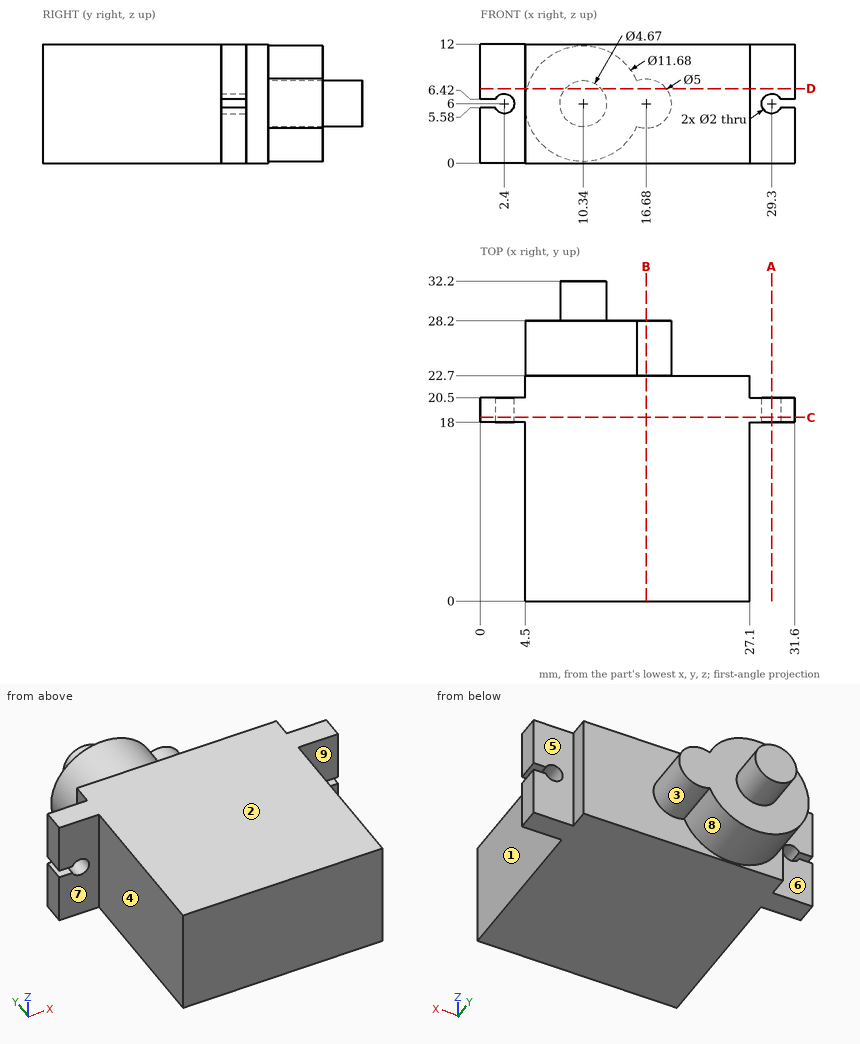
Study the drawing (mm; zero at the part's minimum x, y, z) and answer. A direction names the side the tool comes from. Give positions to 0.01 mm unless a question says otherwise; leave off trailing zeros. Write each loop counter-clockwise with the first axis right and the second up, starting at its lowest first coordinate (ties: lowest second). Pieces come first, ordered by that corner, then holes. Notation, with made-up numbers: (45.25, 76) -> (69.25, 76) arc R22 ccw to (69.25, 97) -> close; hole circle Ø6 at (1, -30.5). An arc over 180 degrees is marked (long way). Write item = value, one per line. Start each with the question number.
1) The part is cut by section A-A, the plane x = 29.3. Determine the outline of the cut face in (y, z).
2) Which of the six approach directions +Z, -Z, +X, -X, +Y, -Y give full straight-line access (tool end or side, diameter ignored) to the marked faces 5, 6, 7, 8 and 9?
3) The part is cut by section D-D, the plane z = 7.5. Determine the outline of the cut face in (x, y), and give its area (3 significant figures).
4) The part is cut by section C-C, the plane y = 18.5. Determine the outline of the cut face in (x, z).
5) The part is cut by section B-B, the plane x = 16.68. Determine the outline of the cut face in (y, z).
6) Determine the mould class of the marked faces 1, 2, 3 and 4 for opening direction X: +X half, -X half, draft (parallel to the pull), parting line (faces both ways), or undercut.
7) Straight lines are drawn through the part: line 1 along Z through (x, y) = (2.4, 18.8); line 2 along Y through (x, z) = (18.5, 5.5); line 3 along X through (y, z) = (2, 5.75). For each, find the intervals that lie inside material, in ascending order.
8) Each of these flat-tipped pins is pushed along its axis until it touches: pin 1 (2 mm diameter, centred on y = 25.5, z = 4.5, fed in from +X); pin 2 (2 mm diameter, centred on x = 2.5, z = 3.5, fed in from +Y); pin 3 (3 mm diameter, centred on y = 9.5, z = 10, fed in from +X); pin 4 (1.6 mm diameter, centred on x = 29.3, z = 6, fed in from -Y). Where does it stop, or does it pass through?
Solutions:
q1.outline = (18, 0) -> (20.5, 0) -> (20.5, 5) -> (18, 5) -> close; (18, 7) -> (20.5, 7) -> (20.5, 12) -> (18, 12) -> close
q2.face_5 = +Z, -Z, +X, +Y
q2.face_6 = +Z, -Z, -X, +Y
q2.face_7 = +Z, -Z, -X, -Y
q2.face_8 = +Y
q2.face_9 = +Z, -Z, +X, -Y
q3.outline = (0, 18) -> (4.5, 18) -> (4.5, 0) -> (27.1, 0) -> (27.1, 18) -> (31.6, 18) -> (31.6, 20.5) -> (27.1, 20.5) -> (27.1, 22.7) -> (18.68, 22.7) -> (18.68, 28.2) -> (12.13, 28.2) -> (12.13, 32.2) -> (8.55, 32.2) -> (8.55, 28.2) -> (4.7, 28.2) -> (4.7, 22.7) -> (4.5, 22.7) -> (4.5, 20.5) -> (0, 20.5) -> close
q3.area = 627 mm²
q4.outline = (0, 0) -> (31.6, 0) -> (31.6, 5.58) -> (30.21, 5.58) arc R1 cw (long way) to (30.21, 6.42) -> (31.6, 6.42) -> (31.6, 12) -> (0, 12) -> (0, 6.42) -> (1.49, 6.42) arc R1 cw (long way) to (1.49, 5.58) -> (0, 5.58) -> close
q5.outline = (0, 0) -> (22.7, 0) -> (22.7, 3.5) -> (28.2, 3.5) -> (28.2, 8.5) -> (22.7, 8.5) -> (22.7, 12) -> (0, 12) -> close
q6.face_1 = +X half
q6.face_2 = draft
q6.face_3 = undercut
q6.face_4 = -X half
q7.line_1 = 0 to 5, 7 to 12
q7.line_2 = 0 to 28.2
q7.line_3 = 4.5 to 27.1
q8.pin_1 = 19.13
q8.pin_2 = 20.5
q8.pin_3 = 27.1
q8.pin_4 = through
